Part print with two shaded views. Sizes in mm from the minimum x, y, z corner. A direction names the side the tool comes from. Give positions to 0.01 mm unless a question says otherwise; leave off trailing zeros. Write each loop counter-clockwise with the first axis right and the second up, starting at its lowest first coordinate (ties: lowest second). Pieces come first, ordered by that corner, then holes.
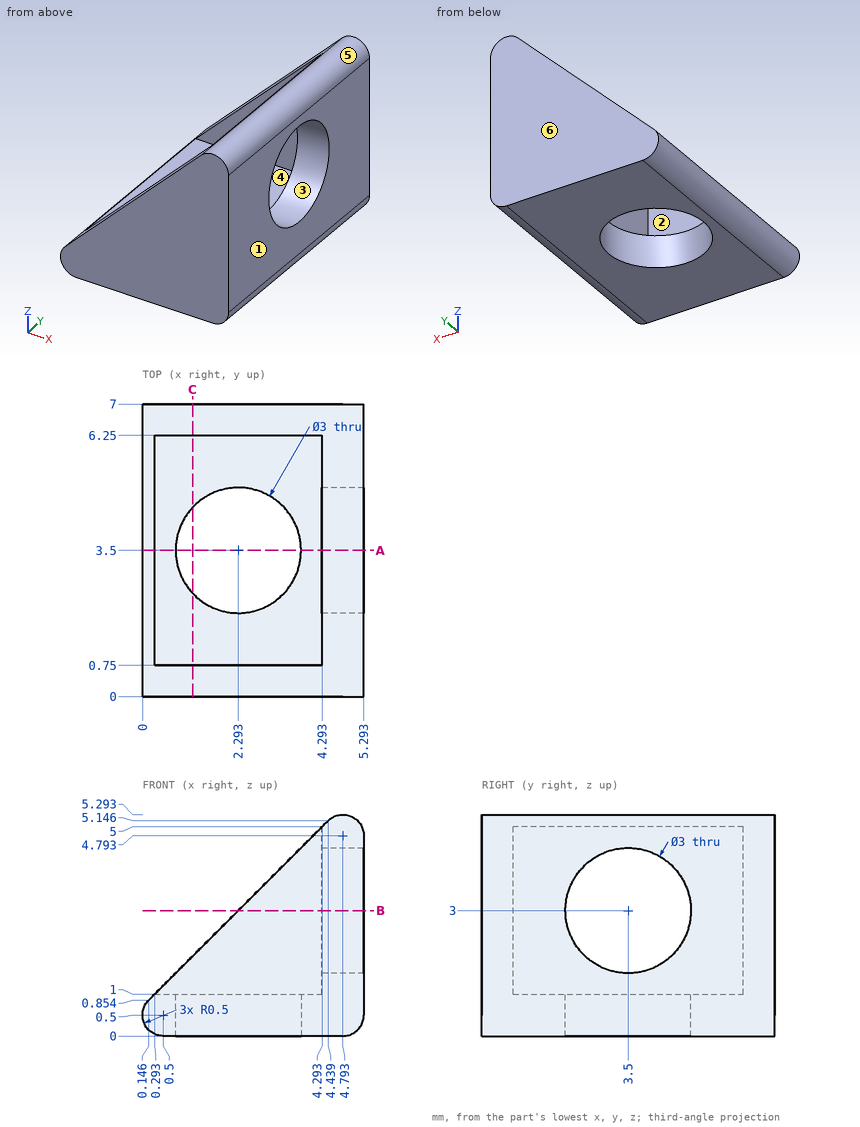
1) Drill centre lines: L1, parallel to Y at x = 3.95, z = 4.1; L2, parallel to X at y = 5, z = 4.5; L3, parallel to Z at x = 4.7, y = 2.75 (1 decimal). Where is each one in solid material? Low to high.
Check result:
L1: y = 0 to 0.75, 6.25 to 7
L2: x = 4.29 to 5.29
L3: z = 0 to 1.7, 4.3 to 5.3
2) Saw through at B-B (z = 3). Write the cut outline in (x, y).
Check result:
outline: (2.29, 0) - (5.29, 0) - (5.29, 2) - (4.29, 2) - (4.29, 0.75) - (2.29, 0.75) - close; (2.29, 6.25) - (4.29, 6.25) - (4.29, 5) - (5.29, 5) - (5.29, 7) - (2.29, 7) - close
3) Saw through at A-A (y = 3.5). Write the cut outline in (x, z).
Check result:
outline: (0.15, 0.85) arc R0.5 ccw to (0.5, 0) - (0.79, 0) - (0.79, 1) - (0.29, 1) - close; (3.79, 0) - (4.79, 0) arc R0.5 ccw to (5.29, 0.5) - (5.29, 1.5) - (4.29, 1.5) - (4.29, 1) - (3.79, 1) - close; (4.29, 4.5) - (5.29, 4.5) - (5.29, 4.79) arc R0.5 ccw to (4.44, 5.15) - (4.29, 5) - close
4) 3-axis set-ups, long thin cutter, end or side, ignore diameter. For the marked faces 1 and 2: which of +Z, -Z, +X, -X, +Y, -Y reach the whole face in a straight line?
Check result:
face 1: +Z, -Z, +X, +Y, -Y
face 2: +Z, -X
5) Flat gauge pins, fed straight in: P1, Ø2.5, axis at x = 2.29, y = 3.5, coming from the +Z side; P2, Ø3, axis at y = 4.5, z = 3.5, coming from the -X side. Where does each tip first touch, or does it go through?
Check result:
P1: passes through
P2: stops at x = 4.29
6) Saw through at C-C (x = 1.2). Write the cut outline in (y, z).
Check result:
outline: (0, 0) - (2.47, 0) - (2.47, 1) - (0.75, 1) - (0.75, 1.91) - (0, 1.91) - close; (4.53, 0) - (7, 0) - (7, 1.91) - (6.25, 1.91) - (6.25, 1) - (4.53, 1) - close
7) Mould opens along Y. For the marked faces 3, 4, 5 and 6 say: +Y half, -Y half, draft (parallel to the pull), parting line (faces both ways), or undercut.
Check result:
face 3: undercut
face 4: undercut
face 5: draft
face 6: +Y half
